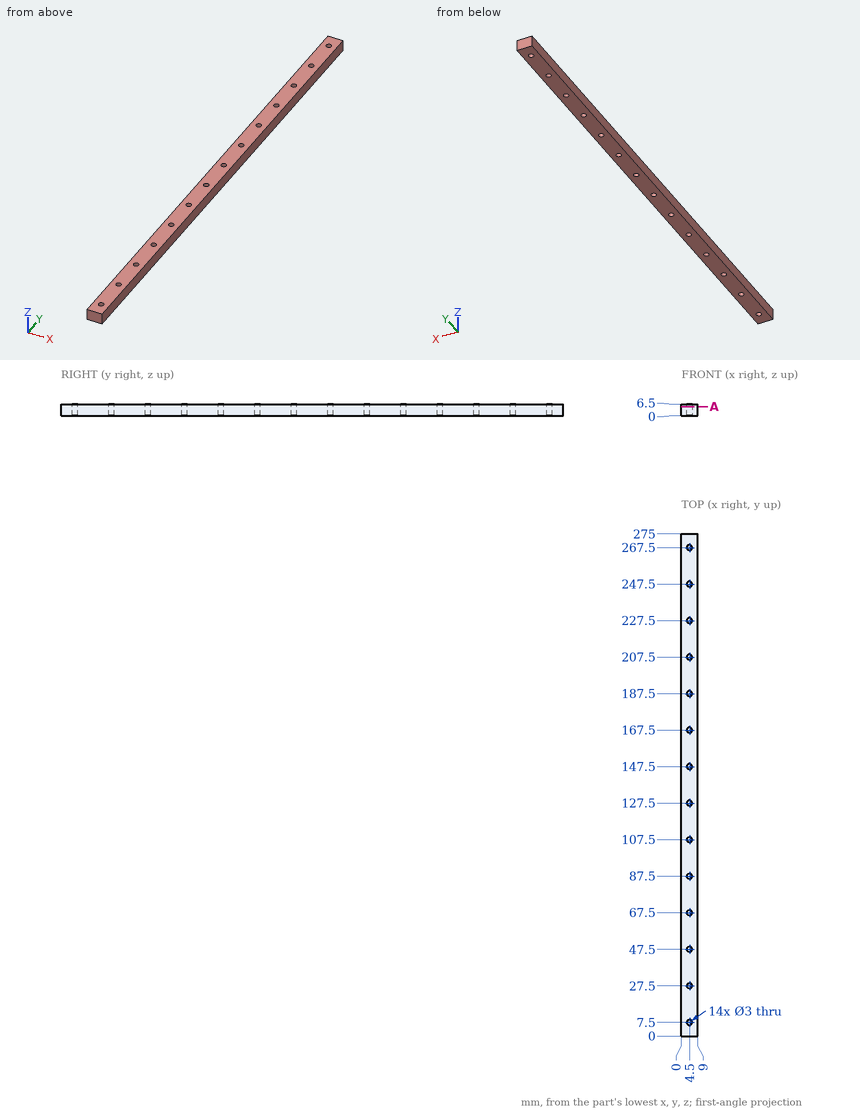
Job drawing, mm, ordinate dimensions from the low corner. One solid piece. Give positions to 0.01 mm unless a question says otherwise; leave off trailing zeros. Return JSON: item names as keys, results as strings.
Q1. Flat gauge pin, fed straight in: pin 1 (1.8 mm diameter, centred on x = 4.5, y = 187.5, fed in from +Z). Where does the tip first touch, or does it go through?
Answer list:
{"pin 1": "passes through"}
Q2. Wall check: probe 1 along X at (y, z) = (87.5, 4.5); probe 2 along X at (y, z) = (46.5, 3.5). Give the ranges that are in metal, low to high. Write a range as from..to.
Answer list:
{"probe 1": "x = 0..3, 6..9", "probe 2": "x = 0..3.38, 5.62..9"}
Q3. Band-saw the part on A-A (z = 5). Count the separate pieces of the cut face and the enclosed holes in it, then the cut area to 3 significant figures.
Answer list:
{"separate pieces": "1", "enclosed holes": "14", "area": "2,380 mm^2"}
